For this review, take the finished solid that the model builds, in its own axes (mm). Face numbers are marked on the shaded views. Round coordinates to 2 decimals unless told otherwise and drop trailing zeros. Loops run counter-clockwise (first coordinate to the right, second up) from the corner with the lowest first, then second, coordinate; pieces in that order, holes last. Notation, with made-up numbers: (-27.75, 73) -> (-3.75, 73) arc R25 ccw to (-3.75, 96) -> close; hole circle Ø7 at (-11, 48). An arc over 180 degrees is marked (long way). Write each question's results on one line, items separated by ' | '.
```python
from build123d import *

# Parameters (mm, degrees)
SKETCH3_W           = 101.6
SKETCH3_H           = 101.6
SHELL2_T            = -2.54
SKETCH8_W           = 95.49459984
SKETCH8_H           = 95.49459984
BOSS_EXTRUDE1_DEPTH = 2.54
SKETCH9_R           = 5.715
CUT_EXTRUDE1_DEPTH  = 2.54


with BuildPart() as part:
    # Sketch3 → Loft1 section 0
    with BuildSketch(Plane(origin=(0, 0, 0), x_dir=(1, 0, 0), z_dir=(0, 1, 0)), mode=Mode.PRIVATE) as loft1_s0:
        Rectangle(SKETCH3_W, SKETCH3_H)
    loft([Vertex(0, 76.2, 0), loft1_s0.sketch])

    # Shell2
    shell2_openings = [part.faces().sort_by_distance(p)[0] for p in [
        (0, 0, 0),
    ]]
    offset(amount=SHELL2_T, openings=shell2_openings, kind=Kind.INTERSECTION)

    # Sketch8 → Boss-Extrude1 (add)
    with BuildSketch(Plane.XZ):
        Rectangle(SKETCH8_W, SKETCH8_H)
    extrude(amount=-BOSS_EXTRUDE1_DEPTH)

    # Sketch9 → Cut-Extrude1 (cut)
    with BuildSketch(Plane(origin=(0, 23.446153846, -35.169230769), x_dir=(-1, 0, 0), z_dir=(0, 0.554700196, -0.832050294))):
        with Locations((35.4584, -19.288769968)):
            Circle(SKETCH9_R)
    extrude(amount=-CUT_EXTRUDE1_DEPTH, mode=Mode.SUBTRACT)


solid = part.part
```
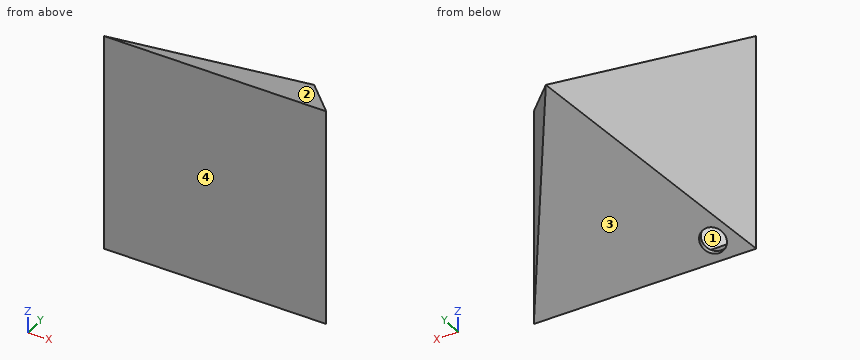
1. Consider section A-A (x = -24). State the section outline as (y, z) points.
Values found:
outline: (0, -50.8) -> (40.2, -24) -> (40.2, 24) -> (0, 50.8) -> close; hole (2.54, -46.05) -> (35.62, -24) -> (35.62, 24) -> (2.54, 46.05) -> close
2. For pin 1 (1 mm diameter, centred on x = -24, z = -27, fed in from +Y); pin 2 (1.5 mm diameter, centred on y = 27.5, z = 9.5, fed in from -X); pin 3 (5 mm diameter, centred on x = 11.5, y = 61.5, fed in from -Z), all flat-tipped, find the tip position at first contact; note any pin that passes through.
Values found:
pin 1: stops at y = 36.45 | pin 2: stops at x = -32.97 | pin 3: stops at z = -11.47
3. Consider section B-B (y = 64). State the section outline as (x, z) points, plus the area to 3 significant figures.
Values found:
outline: (-8.13, -8.13) -> (8.13, -8.13) -> (8.13, 8.13) -> (-8.13, 8.13) -> close; hole (-5.08, -5.08) -> (5.08, -5.08) -> (5.08, 5.08) -> (-5.08, 5.08) -> close | area: 161 mm2
4. Consider section C-C (x = -34.5). State the section outline as (y, z) points.
Values found:
outline: (0, -50.8) -> (2.71, -48.99) -> (1.3, -46.88) -> (2.54, -46.05) -> (2.54, 46.05) -> (19.87, 34.5) -> (19.87, -34.5) -> (10.68, -40.63) -> (12.08, -42.74) -> (24.45, -34.5) -> (24.45, 34.5) -> (0, 50.8) -> close
5. Draft analysis for pull direction Z (two halves, no side actions). For the marked faces 1, 2, 3 and 4, state which applies: released by +Z, released by -Z, zero draft, split by the parting line, or undercut.
Values found:
face 1: undercut | face 2: released by +Z | face 3: released by -Z | face 4: zero draft
6. To check wall thickness, follow probe 1 along Z at (x, y) = (17, 44); probe 2 along Y at (x, z) = (43, -15); probe 3 along X at (y, z) = (49.5, -2.5). State the ranges of each line that lie inside material, in increasing order.
Values found:
probe 1: z = -21.47 to -18.41, 18.41 to 21.47 | probe 2: y = 0 to 2.54, 7.12 to 11.7 | probe 3: x = -17.8 to -14.75, 14.75 to 17.8
